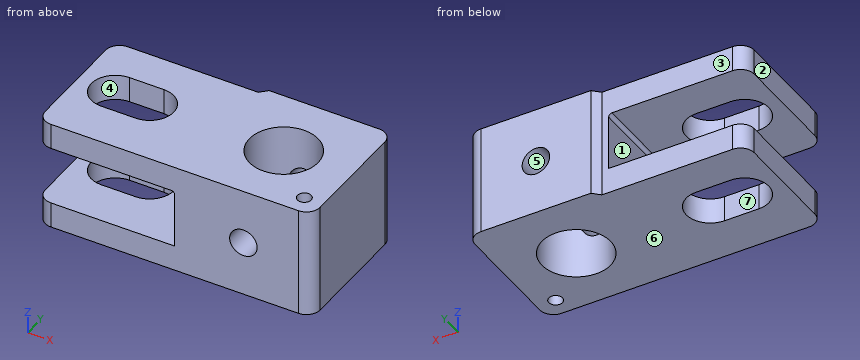
from build123d import *

# Parameters (mm, degrees)
SKETCH_1_R          = 5
EXTRUDE_1_DEPTH     = 8
CHAMFER_1_SIZE      = 1
FILLET_1_R          = 2
SKETCH_2_W          = 20
SKETCH_2_H          = 8.5
CUT_EXTRUDE_1_DEPTH = 37.400549446
SKETCH_3_R          = 1
CUT_EXTRUDE_2_DEPTH = 36.440090293
FILLET_2_R          = 0.5
SKETCH_4_R          = 2
CUT_EXTRUDE_3_DEPTH = 37.932370625


with BuildPart() as part:
    # 草图1 → 凸台-拉伸1 (new, symmetric)
    with BuildSketch(Plane.XY):
        Polygon((-10, -10), (10, -10), (10, 10), (-8, 10), (-8, 9), (-10, 9), (-30, 9), (-30, -10), align=None)
        Circle(SKETCH_1_R, mode=Mode.SUBTRACT)
        with BuildLine():
            Line((-24.5, 3.5), (-19.5, 3.5))
            ThreePointArc((-19.5, 3.5), (-16, 0), (-19.5, -3.5))
            Line((-19.5, -3.5), (-24.5, -3.5))
            ThreePointArc((-24.5, -3.5), (-28, 0), (-24.5, 3.5))
        make_face(mode=Mode.SUBTRACT)
    extrude(amount=EXTRUDE_1_DEPTH, both=True)

    # 倒角1
    chamfer_1_edges = [part.edges().sort_by_distance(p)[0] for p in [
        (-8, 9, 0),
    ]]
    chamfer(chamfer_1_edges, length=CHAMFER_1_SIZE - 0.0001)  # a hair under: the kernel refuses the full size

    # 圆角1
    fillet_1_edges = [part.edges().sort_by_distance(p)[0] for p in [
        (10, -10, 0),
        (-30, -10, 0),
        (-30, 9, 0),
        (10, 10, 0),
    ]]
    fillet(fillet_1_edges, radius=FILLET_1_R)

    # 草图2 → 切除-拉伸1 (cut, through all)
    with BuildSketch(Plane(origin=(0, 9, 0), x_dir=(1, 0, 0), z_dir=(0, 1, 0))):
        with Locations((-20, 0)):
            Rectangle(SKETCH_2_W, SKETCH_2_H)
    extrude(amount=-CUT_EXTRUDE_1_DEPTH, mode=Mode.SUBTRACT)

    # 草图3 → 切除-拉伸2 (cut, through all)
    with BuildSketch(Plane.XY.offset(8)):
        with Locations((7.25, -7.25)):
            Circle(SKETCH_3_R)
    extrude(amount=-CUT_EXTRUDE_2_DEPTH, mode=Mode.SUBTRACT)

    # 圆角2
    fillet_2_edges = [part.edges().sort_by_distance(p)[0] for p in [
        (-10, -0.5, 4.25),
    ]]
    fillet(fillet_2_edges, radius=FILLET_2_R)

    # 草图4 → 切除-拉伸3 (cut, through all)
    with BuildSketch(Plane(origin=(0, 10, 0), x_dir=(1, 0, 0), z_dir=(0, 1, 0))):
        with Locations(Location((0, 0, 0), (0, 0, 180))):
            Circle(SKETCH_4_R)
    extrude(amount=-CUT_EXTRUDE_3_DEPTH, mode=Mode.SUBTRACT)


solid = part.part
Check sheet for the modelled part. Datum: model origin and axes. Units: mm. Face numbers are marked on the shaded views. A direction names the side the tool comes from. Round coordinates to 2 decimals unless told otherwise and drop trailing zeros. Loops run counter-clockwise (first coordinate to the right, second up) from the corner with the lowest first, then second, coordinate; pieces in that order, holes last.
1. Set-up check for the marked faces 1, 2, 3 and 4: record each of +Z, -Z, +X, -X, +Y, -Y from which the full face is reachable in a straight line by a thin tool's end or side.
2. Sectioned sample at C-C on x = 7.25. Record the boundary of the cut face in (y, z), and give its area (3 significant figures).
3. Sectioned sample at D-D on y = 0. Record the boundary of the cut face in (x, z), and give its area (3 significant figures).
4. Mould release check, pull along Z, two halves, no side actions. Record for the marked faces 5, 6 and 7: released by +Z, released by -Z, zero draft, split by the parting line, or undercut.
5. Gauge pin test, flat ends, axial feed: pin 1 Ø4 at (y, z) = (1, 0) entering from -X; pin 2 Ø3 at (x, z) = (-21.5, 6.5) entering from +Y. Record the tip position at first contact, or that the pin passes through.
6. Scan lines: probe 1 along X at (y, z) = (-0.25, -4.75); probe 2 along Z at (x, y) = (-12, -6.25); probe 3 along Z at (x, y) = (0, 8.6). Record each from-to range of solid material in increasing order.
7. Sectioned sample at B-B on z = 0. Give the number of separate pieces and of enclosed holes in the cut face, and give its area (3 significant figures).
8. Sectioned sample at A-A on y = -7.25. Record the boundary of the cut face in (x, z), and give its area (3 significant figures).
Recorded:
1. face 1: -X, +Y, -Y
1. face 2: +Z, -Z, -X, +Y, -Y
1. face 3: +Z, -Z, -X, +Y
1. face 4: +Z, -Z
2. outline: (-10, -8) - (-8.25, -8) - (-8.25, 8) - (-10, 8) - close; (-6.25, -8) - (10, -8) - (10, 8) - (-6.25, 8) - close
2. area: 288 mm2
3. outline: (-30, -8) - (-28, -8) - (-28, -4.25) - (-30, -4.25) - close; (-30, 4.25) - (-28, 4.25) - (-28, 8) - (-30, 8) - close; (-16, -8) - (-5, -8) - (-5, 8) - (-16, 8) - (-16, 4.25) - (-10.5, 4.25) arc R0.5 cw to (-10, 3.75) - (-10, -4.25) - (-16, -4.25) - close; (5, -8) - (10, -8) - (10, 8) - (5, 8) - close
3. area: 220 mm2
4. face 5: undercut
4. face 6: released by -Z
4. face 7: zero draft
5. pin 1: stops at x = -10
5. pin 2: stops at y = 9
6. probe 1: x = -30 to -27.99, -16.01 to -4.99, 4.99 to 10
6. probe 2: z = -8 to -4.25, 4.25 to 8
6. probe 3: z = -8 to -2, 2 to 8
7. separate pieces: 2
7. enclosed holes: 1
7. area: 274 mm2
8. outline: (-30, -8) - (6.25, -8) - (6.25, 8) - (-30, 8) - (-30, 4.25) - (-10.5, 4.25) arc R0.5 cw to (-10, 3.75) - (-10, -4.25) - (-30, -4.25) - close; (8.25, -8) - (10, -8) - (10, 8) - (8.25, 8) - close; hole circle Ø4 at (0, 0)
8. area: 425 mm2
